from build123d import *

# Parameters (mm, degrees)
SKETCH_1_R      = 5
EXTRUDE_1_DEPTH = 18
SKETCH_2_R      = 10
EXTRUDE_2_DEPTH = 8
SKETCH_3D_1_R   = 4


with BuildPart() as part:
    # 草圖1 → 填料-伸長1 (new body)
    with BuildSketch(Plane(origin=(0, 0, 0), x_dir=(1, 0, 0), z_dir=(0, 1, 0))):
        with Locations(Location((0, 0, 0), (0, 0, 270))):
            Circle(SKETCH_1_R)
    extrude(amount=EXTRUDE_1_DEPTH)

    # 草圖2 → 填料-伸長2 (add)
    with BuildSketch(Plane(origin=(0, 18, 0), x_dir=(1, 0, 0), z_dir=(0, 1, 0))):
        with Locations(Location((0, 0, 0), (0, 0, 270))):
            Circle(SKETCH_2_R)
    extrude(amount=EXTRUDE_2_DEPTH)

    # Sketch 3D_1 → 旋轉1 (revolve)
    with BuildSketch(Plane(origin=(0, 0, 0), x_dir=(-0.14242880634815436, 0.98980504904867, 0), z_dir=(0, 0, -1)), mode=Mode.PRIVATE) as revolve_1_sk:
        with Locations((21.775711079, 3.13343374)):
            Circle(SKETCH_3D_1_R)
    revolve(revolve_1_sk.sketch.rotate(Axis((0, 38.5, 0), (-1, 0, 0)), 180), axis=Axis((0, 38.5, 0), (-1, 0, 0)))


solid = part.part
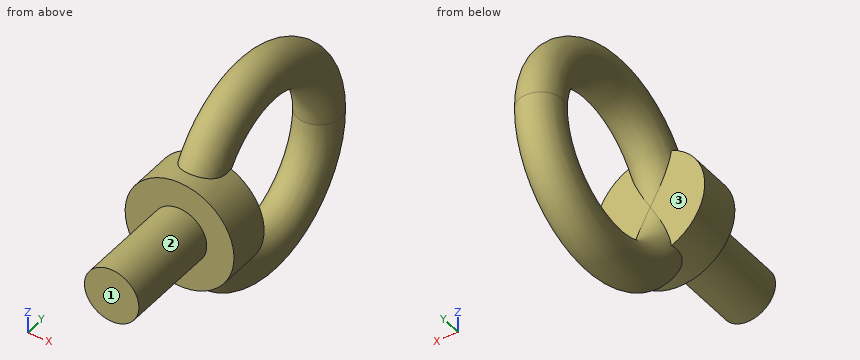
Source: CAD feature listing. Evaluate the final solid. Frame: model axes, mm. Face numbers are marked on the shaded views. Coordinates: 2 decimals unless noted, no trailing zeros. Write each loop counter-clockwise with the first axis right and the second up, starting at its lowest first coordinate (ties: lowest second). Pieces come first, ordered by that corner, then holes. Notation, with made-up numbers: M 44.5,17.25 L 70.5,17.25 A30 cw 70.5,49.25 Z; hole C -25.75,50.25 d8. An arc over 180 degrees is marked long. Use a Markdown table: item, result.
1) Section C-C, the plane x = 6.75. Output: boundary loops of the cut face in (y, z), then the cut area to 3 significant figures.
Conclusion:
| item | result |
|---|---|
| outline | M 18,-7.38 L 26,-7.38 L 26,7.38 L 18,7.38 Z |
| area | 118 mm^2 |
2) Section A-A, the plane x = 3.25. Output: boundary loops of the cut face in (y, z).
Conclusion:
| item | result |
|---|---|
| outline | M 0,-3.8 L 18,-3.8 L 18,-9.46 L 22.22,-9.46 A18.83 ccw long 22.22,9.46 L 18,9.46 L 18,3.8 L 0,3.8 Z; hole M 26,-6.67 A14.17 ccw long 26,6.67 Z |
3) First-contact query: pin 1 Ø8 at (y, z) = (21, 11) entering from -X; pin 2 Ø6 at (x, z) = (3.5, -8.5) entering from +Y; pin 3 Ø12 at (x, z) = (6.5, -11.5) entering from -Y; pin 4 Ø6 at (x, y) = (-7.5, 48) entering from -Z. Flat tips, straight axial feed; report the tip coordinate or a pass-through.
Conclusion:
| item | result |
|---|---|
| pin 1 | stops at x = -7.14 |
| pin 2 | stops at y = 57.73 |
| pin 3 | stops at y = 18 |
| pin 4 | passes through |
4) Ray query, L1, parallel to Y at x = 4.25, z = 7.5; L2, parallel to Z at x = 0.75, y = 42; L3, parallel to Z at x = -0.75, y = 10. Return the intervals inside material, ascending.
Conclusion:
| item | result |
|---|---|
| L1 | y = 18 to 26 |
| L2 | z = -20.13 to -12.07, 12.07 to 20.13 |
| L3 | z = -4.94 to 4.94 |
5) Section B-B, the plane y = 15. Output: boundary loops of the cut face in (x, z).
Conclusion:
| item | result |
|---|---|
| outline | C 0,0 d10 |
6) Mould query, pull axis Y, two halves, no side actions, for the marked faces 1, 2 and 3. Classes: pulls with the +Y half, pulls with the -Y half, needs draft (parallel to the pull), parting line crosses it, or undercut.
Conclusion:
| item | result |
|---|---|
| face 1 | pulls with the -Y half |
| face 2 | needs draft |
| face 3 | undercut |
